Work out the finished part from the listing and answer in its coordinate system (mm). Face numbers are marked on the shaded views. Coordinates: 2 decimals unless noted, no trailing zeros. Order: outer loops, then holes, each group sorted by start corner. A loop starts at its lowest first (then second) coordinate and runs counter-clockwise, first axis right, second up.
1. The part is cut by section A-A, the plane x = 0. Give the vertices of the cut face in (y, z), then the cut area to 3 significant figures.
2. Find the intervals of material crossed by probe 1 along Y at (x, z) = (0, 5.75); probe 2 along X at (y, z) = (-5, 3.5); probe 3 along Y at (x, z) = (0.75, 5), in increasing order.
3. The part is cut by section B-B, the plane y = -4. Give the vertices of the cut face in (x, z), then the cut area to 3 significant figures.
4. A flat-ended cylindrical pin translates along its axis: pin 1 Ø2 at (x, z) = (2, 4) entering from -Y. Find the tip coordinate at first contact, or state that the pin passes through.
5. The part is cut by section D-D, the plane x = -1.15. Give the vertices of the cut face in (y, z), then the cut area to 3 significant figures.
6. Determine the mould class of the marked faces 1, 2, 3 and 4 for opening direction X: +X half, -X half, draft (parallel to the pull), parting line (faces both ways), or undercut.
7. The part is cut by section C-C, the plane z = 5. Give the vertices of the cut face in (x, y).
```python
from build123d import *

# Parameters (mm, degrees)
BOSS_EXTRUDE1_DEPTH      = 8
SCHIZZO1_R               = 1.75
TAGLIO_ESTRUSIONE1_DEPTH = 8


with BuildPart() as part:
    # Sketch1 → Boss-Extrude1 (new body)
    with BuildSketch(Plane.XY):
        with BuildLine():
            Line((-3, 5), (-3, -5))
            ThreePointArc((-3, -5), (0, -8), (3, -5))
            Line((3, -5), (3, 5))
            ThreePointArc((3, 5), (0, 8), (-3, 5))
        make_face()
    extrude(amount=BOSS_EXTRUDE1_DEPTH)

    # Schizzo1 → Taglio-Estrusione1 (cut)
    with BuildSketch(Plane.XY.offset(8)):
        with Locations((0, 5)):
            Circle(SCHIZZO1_R)
    taglio_estrusione1 = extrude(amount=-TAGLIO_ESTRUSIONE1_DEPTH, mode=Mode.SUBTRACT)

    # Specchia1: Taglio-Estrusione1 across plane
    add(taglio_estrusione1.mirror(Plane.ZX), mode=Mode.SUBTRACT)


solid = part.part
```
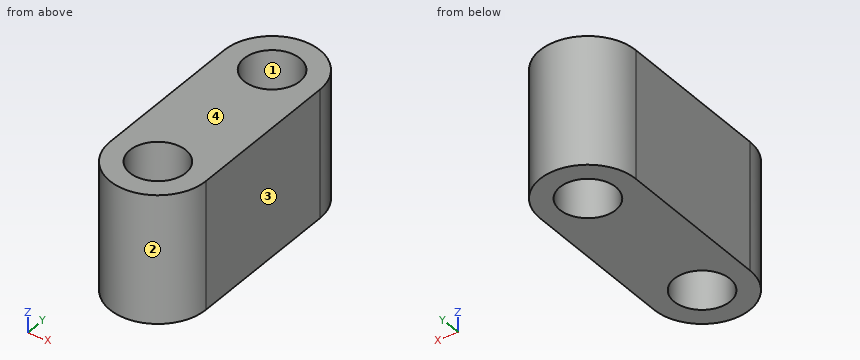
Geometry says:
1. outline: (-8, 0) - (-6.75, 0) - (-6.75, 8) - (-8, 8) - close; (-3.25, 0) - (3.25, 0) - (3.25, 8) - (-3.25, 8) - close; (6.75, 0) - (8, 0) - (8, 8) - (6.75, 8) - close
1. area: 72.0 mm2
2. probe 1: y = -8 to -6.75, -3.25 to 3.25, 6.75 to 8
2. probe 2: x = -3 to -1.75, 1.75 to 3
2. probe 3: y = -7.9 to -6.58, -3.42 to 3.42, 6.58 to 7.9
3. outline: (-3, 0) - (-1.44, 0) - (-1.44, 8) - (-3, 8) - close; (1.44, 0) - (3, 0) - (3, 8) - (1.44, 8) - close
3. area: 25.0 mm2
4. pin 1: stops at y = -7.83
5. outline: (-7.77, 0) - (-6.32, 0) - (-6.32, 8) - (-7.77, 8) - close; (-3.68, 0) - (3.68, 0) - (3.68, 8) - (-3.68, 8) - close; (6.32, 0) - (7.77, 0) - (7.77, 8) - (6.32, 8) - close
5. area: 82.1 mm2
6. face 1: undercut
6. face 2: parting line
6. face 3: +X half
6. face 4: draft
7. outline: (-3, -5) arc R3 ccw to (3, -5) - (3, 5) arc R3 ccw to (-3, 5) - close; hole circle Ø3.5 at (0, -5); hole circle Ø3.5 at (0, 5)
